from build123d import *

# Parameters (mm, degrees)
BOSS_EXTRUDE1_DEPTH = 3
SKETCH2_R           = 2.5
CUT_EXTRUDE1_DEPTH  = 62.822600008
FILLET1_R           = 3


with BuildPart() as part:
    # Sketch1 → Boss-Extrude1 (new body)
    with BuildSketch(Plane(origin=(0, 0, 0), x_dir=(0, 0, -1), z_dir=(1, 0, 0))):
        with BuildLine():
            Line((22.886751346, 10), (30, 10))
            Line((30, 10), (30, -10))
            Line((30, -10), (0, -10))
            ThreePointArc((0, -10), (-5, -8.660254038), (-8.660254038, -5))
            Line((-8.660254038, -5), (-35.103629711, 40.801270189))
            Line((-35.103629711, 40.801270189), (-17.783121635, 50.801270189))
            Line((-17.783121635, 50.801270189), (-2.783121635, 24.820508076))
            ThreePointArc((-2.783121635, 24.820508076), (-1.193935409, 22.749440264), (0.877132403, 21.160254038))
            Line((0.877132403, 21.160254038), (17.886751346, 11.339745962))
            ThreePointArc((17.886751346, 11.339745962), (20.298560895, 10.340741737), (22.886751346, 10))
        make_face()
    extrude(amount=BOSS_EXTRUDE1_DEPTH)

    # Sketch2 → Cut-Extrude1 (cut, through all)
    with BuildSketch(Plane(origin=(3, 0, 0), x_dir=(0, 0, -1), z_dir=(1, 0, 0))):
        with Locations((20.92, 0)):
            Circle(SKETCH2_R)
        with Locations((0.92, 0)):
            Circle(SKETCH2_R)
        with Locations((-14.04, 24.32)):
            Circle(SKETCH2_R)
        with Locations((-21.54, 37.31)):
            Circle(SKETCH2_R)
    extrude(amount=-CUT_EXTRUDE1_DEPTH, mode=Mode.SUBTRACT)

    # Fillet1
    fillet1_edges = [part.edges().sort_by_distance(p)[0] for p in [
        (1.5, 50.801270189, 17.783121635),
        (1.5, 10, -30),
        (1.5, -10, -30),
        (1.5, 40.801270189, 35.103629711),
    ]]
    fillet(fillet1_edges, radius=FILLET1_R)


solid = part.part
Model file for the job. Use its own axes, mm. A direction names the side the tool comes from. Give positions to 0.01 mm unless a question says otherwise; leave off trailing zeros. Loops run counter-clockwise (first coordinate to the right, second up) from the corner with the lowest first, then second, coordinate; pieces in that order, holes last.
1) Flat gauge pins, fed straight in: pin 1 Ø1.5 at (x, z) = (2, 21.5) entering from +Y; pin 2 Ø8 at (y, z) = (0, -0.92) entering from -X; pin 3 Ø1.5 at (x, z) = (1.5, 4) entering from -Y; pin 4 Ø1.5 at (x, z) = (2.5, -1) entering from +Y. Where does each tip first touch, or does it go through?
2) Saw through at D-D (y = 0). Write the cut outline in (x, z), plus the area to 3 significant figures.
3) Saw through at A-A (x = 2.1). Write the cut outline in (y, z).
4) Wall check: line 1 (Z direction, x = 0.75, y = 0.5); line 2 (Y direction, x = 2.7, z = 0.5); line 3 (Y direction, x = 2.05, z = 21.54). Give the ranges that are in metal, low to high.
5) Saw through at B-B (z = 21.54). Write the cut outline in (x, y).
6) Saw through at C-C (y = 37.31). Write the cut outline in (x, z).
7) Tool access for faces 1 (the flat face through (1, 10, -25)), 2 (the cylindrical face through (1.52, 26.43, 12.7)): list every direction of +Z, -Z, +X, -X, +Y, -Y with a clear straight run to the whole face (end or side of a thin tool).
Answer block:
1. pin 1: stops at y = 49.09
1. pin 2: stops at x = 0
1. pin 3: stops at y = -9.46
1. pin 4: stops at y = 21.55
2. outline: (0, -30) - (3, -30) - (3, -23.42) - (0, -23.42) - close; (0, -18.42) - (3, -18.42) - (3, -3.42) - (0, -3.42) - close; (0, 1.58) - (3, 1.58) - (3, 11.55) - (0, 11.55) - close
2. area: 94.6 mm2
3. outline: (-10, -27) arc R3 ccw to (-7, -30) - (7, -30) arc R3 ccw to (10, -27) - (10, -22.89) arc R10 cw to (11.34, -17.89) - (21.16, -0.88) arc R10 cw to (24.82, 2.78) - (48.2, 16.28) arc R3 ccw to (49.3, 20.38) - (42.3, 32.51) arc R3 ccw to (38.2, 33.6) - (-5, 8.66) arc R10 ccw to (-10, 0) - close; hole circle Ø5 at (0, -20.92); hole circle Ø5 at (0, -0.92); hole circle Ø5 at (24.32, 14.04); hole circle Ø5 at (37.31, 21.54)
4. line 1: z = -30 to -23.37, -18.47 to -3.37, 1.53 to 11.84
4. line 2: y = -9.99 to -2.06, 2.06 to 22.12
4. line 3: y = 17.31 to 34.81, 39.81 to 48.63
5. outline: (0, 17.31) - (3, 17.31) - (3, 34.81) - (0, 34.81) - close; (0, 39.81) - (3, 39.81) - (3, 48.63) - (0, 48.63) - close
6. outline: (0, 9.99) - (3, 9.99) - (3, 19.04) - (0, 19.04) - close; (0, 24.04) - (3, 24.04) - (3, 33.09) - (0, 33.09) - close
7. face 1: -Z, +X, -X, +Y
7. face 2: +X, -X
